The listing builds one solid part. Answer for the finished solid, in the listing's coordinates (mm). Coordinates: 2 decimals unless noted, no trailing zeros. Order: outer loops, then holes, each group sorted by start corner. A loop starts at its lowest first (then second) coordinate and runs counter-clockwise, first axis right, second up. Notation, with made-up numbers: (7, 76) -> (49, 76) arc R18 cw to (49, 98) -> close; hole circle Ø2 at (3, 44). An arc over 180 degrees is marked (long way). Answer in a Markdown table with one row per item. Add a question column.
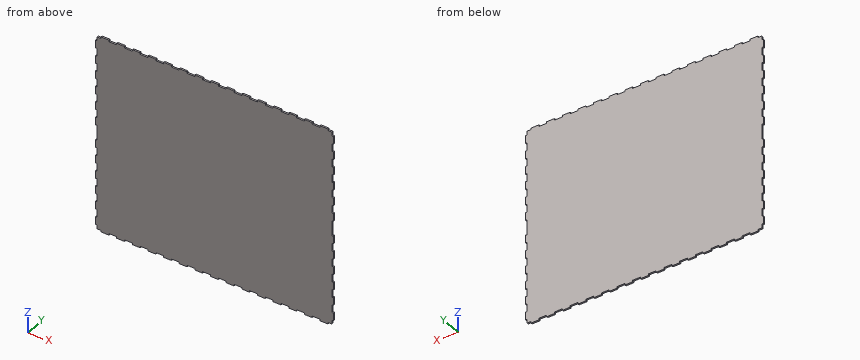
```python
from build123d import *

# Parameters (mm, degrees)
BOSS_EXTRUDE1_DEPTH = 4


with BuildPart() as part:
    # Sketch1 → Boss-Extrude1 (new body)
    with BuildSketch(Plane(origin=(0, 0, 0), x_dir=(1, 0, 0), z_dir=(0, 1, 0))):
        Polygon((9.8625, 250), (-9.8625, 250), (-9.8625, 246), (-29.5875, 246), (-29.5875, 250), (-49.3125, 250), (-49.3125, 246), (-69.0375, 246), (-69.0375, 250), (-88.7625, 250), (-88.7625, 246), (-108.4875, 246), (-108.4875, 250), (-128.2125, 250), (-128.2125, 246), (-147.9375, 246), (-147.9375, 250), (-167.6625, 250), (-167.6625, 246), (-187.3875, 246), (-187.3875, 250), (-207.1125, 250), (-207.1125, 246), (-226.8375, 246), (-226.8375, 250), (-246.5625, 250), (-246.5625, 246), (-266.2875, 246), (-266.2875, 250), (-286.0125, 250), (-286.0125, 246), (-295.8125, 246), (-295.8125, 236.2), (-299.8125, 236.2), (-299.8125, 216.475), (-295.8125, 216.475), (-295.8125, 196.75), (-299.8125, 196.75), (-299.8125, 177.025), (-295.8125, 177.025), (-295.8125, 157.3), (-299.8125, 157.3), (-299.8125, 137.575), (-295.8125, 137.575), (-295.8125, 117.85), (-299.8125, 117.85), (-299.8125, 98.125), (-295.8125, 98.125), (-295.8125, 78.4), (-299.8125, 78.4), (-299.8125, 58.675), (-295.8125, 58.675), (-295.8125, 38.95), (-299.8125, 38.95), (-299.8125, 19.225), (-295.8125, 19.225), (-295.8125, -19.225), (-299.8125, -19.225), (-299.8125, -38.95), (-295.8125, -38.95), (-295.8125, -58.675), (-299.8125, -58.675), (-299.8125, -78.4), (-295.8125, -78.4), (-295.8125, -98.125), (-299.8125, -98.125), (-299.8125, -117.85), (-295.8125, -117.85), (-295.8125, -137.575), (-299.8125, -137.575), (-299.8125, -157.3), (-295.8125, -157.3), (-295.8125, -177.025), (-299.8125, -177.025), (-299.8125, -196.75), (-295.8125, -196.75), (-295.8125, -216.475), (-299.8125, -216.475), (-299.8125, -236.2), (-295.8125, -236.2), (-295.8125, -246), (-286.0125, -246), (-286.0125, -250), (-266.2875, -250), (-266.2875, -246), (-246.5625, -246), (-246.5625, -250), (-226.8375, -250), (-226.8375, -246), (-207.1125, -246), (-207.1125, -250), (-187.3875, -250), (-187.3875, -246), (-167.6625, -246), (-167.6625, -250), (-147.9375, -250), (-147.9375, -246), (-128.2125, -246), (-128.2125, -250), (-108.4875, -250), (-108.4875, -246), (-88.7625, -246), (-88.7625, -250), (-69.0375, -250), (-69.0375, -246), (-49.3125, -246), (-49.3125, -250), (-29.5875, -250), (-29.5875, -246), (-9.8625, -246), (-9.8625, -250), (9.8625, -250), (9.8625, -246), (29.5875, -246), (29.5875, -250), (49.3125, -250), (49.3125, -246), (69.0375, -246), (69.0375, -250), (88.7625, -250), (88.7625, -246), (108.4875, -246), (108.4875, -250), (128.2125, -250), (128.2125, -246), (147.9375, -246), (147.9375, -250), (167.6625, -250), (167.6625, -246), (187.3875, -246), (187.3875, -250), (207.1125, -250), (207.1125, -246), (226.8375, -246), (226.8375, -250), (246.5625, -250), (246.5625, -246), (266.2875, -246), (266.2875, -250), (286.0125, -250), (286.0125, -246), (295.8125, -246), (295.8125, -236.2), (299.8125, -236.2), (299.8125, -216.475), (295.8125, -216.475), (295.8125, -196.75), (299.8125, -196.75), (299.8125, -177.025), (295.8125, -177.025), (295.8125, -157.3), (299.8125, -157.3), (299.8125, -137.575), (295.8125, -137.575), (295.8125, -117.85), (299.8125, -117.85), (299.8125, -98.125), (295.8125, -98.125), (295.8125, -78.4), (299.8125, -78.4), (299.8125, -58.675), (295.8125, -58.675), (295.8125, -38.95), (299.8125, -38.95), (299.8125, -19.225), (295.8125, -19.225), (295.8125, 19.225), (299.8125, 19.225), (299.8125, 38.95), (295.8125, 38.95), (295.8125, 58.675), (299.8125, 58.675), (299.8125, 78.4), (295.8125, 78.4), (295.8125, 98.125), (299.8125, 98.125), (299.8125, 117.85), (295.8125, 117.85), (295.8125, 137.575), (299.8125, 137.575), (299.8125, 157.3), (295.8125, 157.3), (295.8125, 177.025), (299.8125, 177.025), (299.8125, 196.75), (295.8125, 196.75), (295.8125, 216.475), (299.8125, 216.475), (299.8125, 236.2), (295.8125, 236.2), (295.8125, 246), (286.0125, 246), (286.0125, 250), (266.2875, 250), (266.2875, 246), (246.5625, 246), (246.5625, 250), (226.8375, 250), (226.8375, 246), (207.1125, 246), (207.1125, 250), (187.3875, 250), (187.3875, 246), (167.6625, 246), (167.6625, 250), (147.9375, 250), (147.9375, 246), (128.2125, 246), (128.2125, 250), (108.4875, 250), (108.4875, 246), (88.7625, 246), (88.7625, 250), (69.0375, 250), (69.0375, 246), (49.3125, 246), (49.3125, 250), (29.5875, 250), (29.5875, 246), (9.8625, 246), align=None)
    extrude(amount=BOSS_EXTRUDE1_DEPTH)


solid = part.part
```
Q1. A cutting plane is placed at A-A (x = 217.5). Determine the outline of the cut face in (y, z).
Q2. Straight lines are drawn through the part: line 1 (X direction, y = 3.25, z = -89.5); line 2 (Z direction, x = 23.5, y = 3.15). For each, find the intervals that lie inside material, in ascending order.
Q3. Given pin 1 (2 mm diameter, centred on x = -297, y = 2, fed in from -Z); pin 2 (1.2 mm diameter, centred on y = 1.5, z = -247.5, fed in from -X); pin 3 (2 mm diameter, centred on x = 293, y = 2.5, fed in from -Z), each flat-ended and moving along its own axis, determine where each tip first touches the part or whether it passes through.
Returned:
| question | item | result |
|---|---|---|
| 1 | outline | (0, -246) -> (4, -246) -> (4, 246) -> (0, 246) -> close |
| 2 | line 1 | x = -295.81 to 295.81 |
| 2 | line 2 | z = -246 to 246 |
| 3 | pin 1 | stops at z = -236.2 |
| 3 | pin 2 | stops at x = -286.01 |
| 3 | pin 3 | stops at z = -246 |
